Could you check a few things on this model? Use its own coordinates, in mm. Face numbers are marked on the shaded views. A direction names the side the tool comes from. Round coordinates to 2 decimals unless told otherwise and drop trailing zeros. Loops run counter-clockwise (first coordinate to the right, second up) from the corner with the lowest first, then second, coordinate; pieces in that order, holes last.
from build123d import *

# Parameters (mm, degrees)
SKETCH1_R           = 27
BOSS_EXTRUDE1_DEPTH = 95
SKETCH2_R           = 26
BOSS_EXTRUDE2_DEPTH = 99.5
SKETCH3_R           = 16
BOSS_EXTRUDE3_DEPTH = 3
SKETCH4_R           = 6
BOSS_EXTRUDE4_DEPTH = 22
CUT_EXTRUDE1_DEPTH  = 15
SKETCH6_R           = 2.5
CUT_EXTRUDE2_DEPTH  = 10
SKETCH7_R           = 26
BOSS_EXTRUDE5_DEPTH = 18


with BuildPart() as part:
    # Sketch1 → Boss-Extrude1 (new body)
    with BuildSketch(Plane(origin=(0, 0, 0), x_dir=(1, 0, 0), z_dir=(0, 1, 0))):
        Circle(SKETCH1_R)
    extrude(amount=BOSS_EXTRUDE1_DEPTH)

    # Sketch2 → Boss-Extrude2 (add)
    with BuildSketch(Plane(origin=(0, 95, 0), x_dir=(1, 0, 0), z_dir=(0, 1, 0))):
        Circle(SKETCH2_R)
    extrude(amount=BOSS_EXTRUDE2_DEPTH)

    # Sketch3 → Boss-Extrude3 (add)
    with BuildSketch(Plane(origin=(0, 194.5, 0), x_dir=(1, 0, 0), z_dir=(0, 1, 0))):
        Circle(SKETCH3_R)
    extrude(amount=BOSS_EXTRUDE3_DEPTH)

    # Sketch4 → Boss-Extrude4 (add)
    with BuildSketch(Plane(origin=(0, 197.5, 0), x_dir=(1, 0, 0), z_dir=(0, 1, 0))):
        Circle(SKETCH4_R)
    extrude(amount=BOSS_EXTRUDE4_DEPTH)

    # Sketch5 → Cut-Extrude1 (cut)
    with BuildSketch(Plane(origin=(0, 219.5, 0), x_dir=(1, 0, 0), z_dir=(0, 1, 0))):
        with BuildLine():
            Line((-4.472135955, 4), (4.472135955, 4))
            ThreePointArc((4.472135955, 4), (0, 6), (-4.472135955, 4))
        make_face()
    extrude(amount=-CUT_EXTRUDE1_DEPTH, mode=Mode.SUBTRACT)

    # Sketch6 → Cut-Extrude2 (cut)
    with BuildSketch(Plane(origin=(0, 194.5, 0), x_dir=(1, 0, 0), z_dir=(0, 1, 0))):
        with Locations((0, 20)):
            Circle(SKETCH6_R)
        with Locations((-20, 0)):
            Circle(SKETCH6_R)
        with Locations((0, -20)):
            Circle(SKETCH6_R)
        with Locations((20, 0)):
            Circle(SKETCH6_R)
    extrude(amount=-CUT_EXTRUDE2_DEPTH, mode=Mode.SUBTRACT)

    # Sketch7 → Boss-Extrude5 (add)
    with BuildSketch(Plane.XZ):
        Circle(SKETCH7_R)
    extrude(amount=BOSS_EXTRUDE5_DEPTH)


solid = part.part
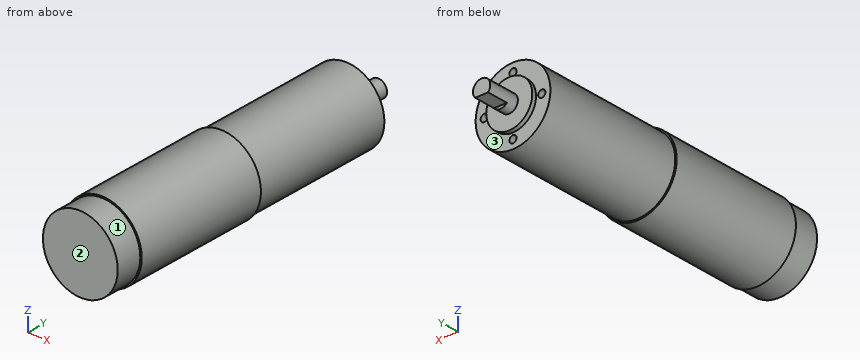
Item 1: If we section it at B-B, the plane z = 0: Please give me the cut outline in (x, y), then the cut area to 3 significant figures.
Results list:
outline: (-27, 0) - (-26, 0) - (-26, -18) - (26, -18) - (26, 0) - (27, 0) - (27, 95) - (26, 95) - (26, 194.5) - (22.5, 194.5) - (22.5, 184.5) - (17.5, 184.5) - (17.5, 194.5) - (16, 194.5) - (16, 197.5) - (6, 197.5) - (6, 219.5) - (-6, 219.5) - (-6, 197.5) - (-16, 197.5) - (-16, 194.5) - (-17.5, 194.5) - (-17.5, 184.5) - (-22.5, 184.5) - (-22.5, 194.5) - (-26, 194.5) - (-26, 95) - (-27, 95) - close
area: 11,500 mm2
Item 2: Will these pins go through, and if not, where does the flat tip stop? pin 1 (2 mm diameter, centred on x = -9, z = 16.5, fed in from +Y); pin 2 (1.6 mm diameter, centred on x = -1, z = -5.5, fed in from +Y); pin 3 (2.5 mm diameter, centred on x = 0.5, z = -19.5, fed in from +Y).
Results list:
pin 1: stops at y = 194.5
pin 2: stops at y = 204.5
pin 3: stops at y = 184.5
Item 3: If we section it at C-C, the plane y = 128: Please give me the cut outline in (x, z), then the cut area to 3 significant figures.
Results list:
outline: circle Ø52 at (0, 0)
area: 2,120 mm2
Item 4: For the marked faces 1, 2 and 3, which set-ups out of +Z, -Z, +X, -X, +Y, -Y let a thin tool reach every point of the face, with its end or its side?
Results list:
face 1: -Y
face 2: +Z, -Z, +X, -X, -Y
face 3: +Y
Item 5: If I drill on line 1 along X through (y, z) = (187, 0); line 2 along Y through (x, z) = (-2.5, -21.5), over which ranges is the centre line in solid material (lowest first)?
Results list:
line 1: x = -26 to -22.5, -17.5 to 17.5, 22.5 to 26
line 2: y = -18 to 194.5
Item 6: If we section it at D-D, the plane z = -20: Please give me the cut outline in (x, y), then the cut area to 3 significant figures.
Results list:
outline: (-18.14, 0) - (-16.61, 0) - (-16.61, -18) - (16.61, -18) - (16.61, 0) - (18.14, 0) - (18.14, 95) - (16.61, 95) - (16.61, 194.5) - (2.5, 194.5) - (2.5, 184.5) - (-2.5, 184.5) - (-2.5, 194.5) - (-16.61, 194.5) - (-16.61, 95) - (-18.14, 95) - close
area: 7,300 mm2
